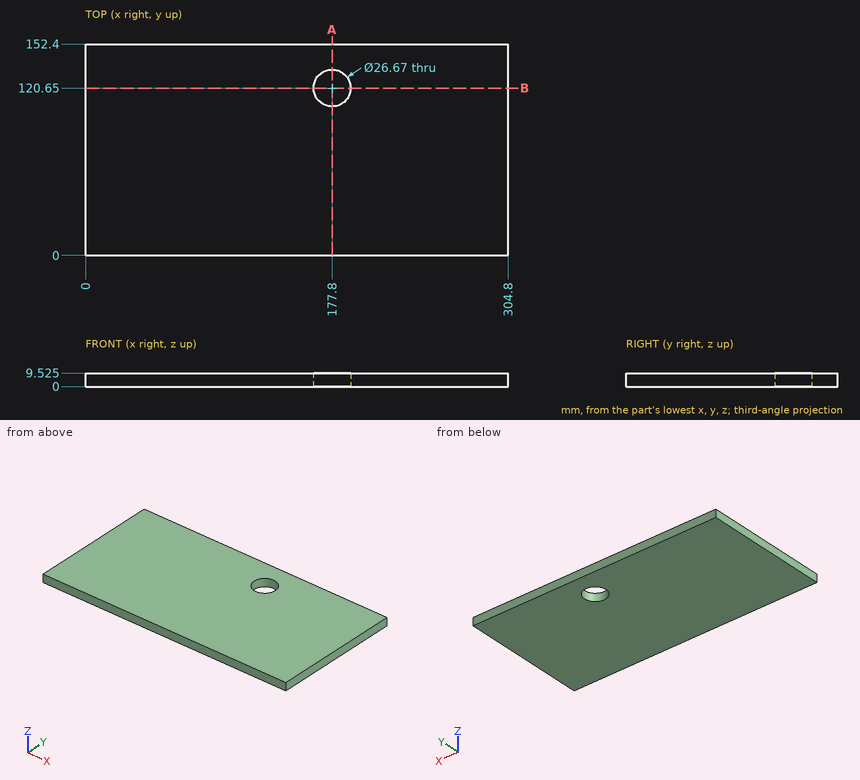
Check sheet for the drawn part. Datum: minimum x, y, z corner. Units: mm. Coordinates: 2 decimals unless noted, no trailing zeros. Loops run counter-clockwise (first coordinate to the right, second up) from the corner with the lowest first, then second, coordinate; pieces in that order, holes last. Notation, with made-up numbers: (40.5, -24) -> (85.5, -24) arc R26 cw to (85.5, 3) -> close; hole circle Ø3 at (29.5, 67.25). An arc over 180 degrees is marked (long way). Answer in a Markdown table with one row per item.
1. Sectioned sample at A-A, the plane x = 177.8. Record the boundary of the cut face in (y, z) (3 decimals).
Check values:
| item | result |
|---|---|
| outline | (0, 0) -> (107.315, 0) -> (107.315, 9.525) -> (0, 9.525) -> close; (133.985, 0) -> (152.4, 0) -> (152.4, 9.525) -> (133.985, 9.525) -> close |
2. Sectioned sample at B-B, the plane y = 120.65. Record the boundary of the cut face in (x, z) (3 decimals).
Check values:
| item | result |
|---|---|
| outline | (0, 0) -> (164.465, 0) -> (164.465, 9.525) -> (0, 9.525) -> close; (191.135, 0) -> (304.8, 0) -> (304.8, 9.525) -> (191.135, 9.525) -> close |
3. Go/stop test with flat-tipped pins: pin 1 (16 mm diameter, centred on x = 177.8, y = 120.65, fed in from -Z); pin 2 (12 mm diameter, centred on x = 39, y = 111.5, fed in from -Z). Record where each tip stops, or that it passes through.
Check values:
| item | result |
|---|---|
| pin 1 | passes through |
| pin 2 | stops at z = 0 |
4. Material ranges on line 1 along Y through (x, z) = (177.8, 4.25) (3 decimals); line 2 along X through (y, z) = (128, 3), recorded low to high. Write a range as [from, to].
Check values:
| item | result |
|---|---|
| line 1 | y = [0, 107.315], [133.985, 152.4] |
| line 2 | x = [0, 166.67], [188.93, 304.8] |
